Answer from the drawing. Dimensions are ordinates in mm from the lowest x, y and z of the part. Give positions to 0.01 mm unless a question says otherwise; leave off trailing zeros. Loops run counter-clockwise (first coordinate to the right, second up) from the corner with the lowest first, then second, coordinate; pieces in that order, holes last. Notation, with made-up numbers: M 26,-32 L 53,-32 A10 cw 53,-25 Z; hole C -1.75,-36.5 d10. An arc over 180 degrees is marked long. Use a Markdown table: item, result.
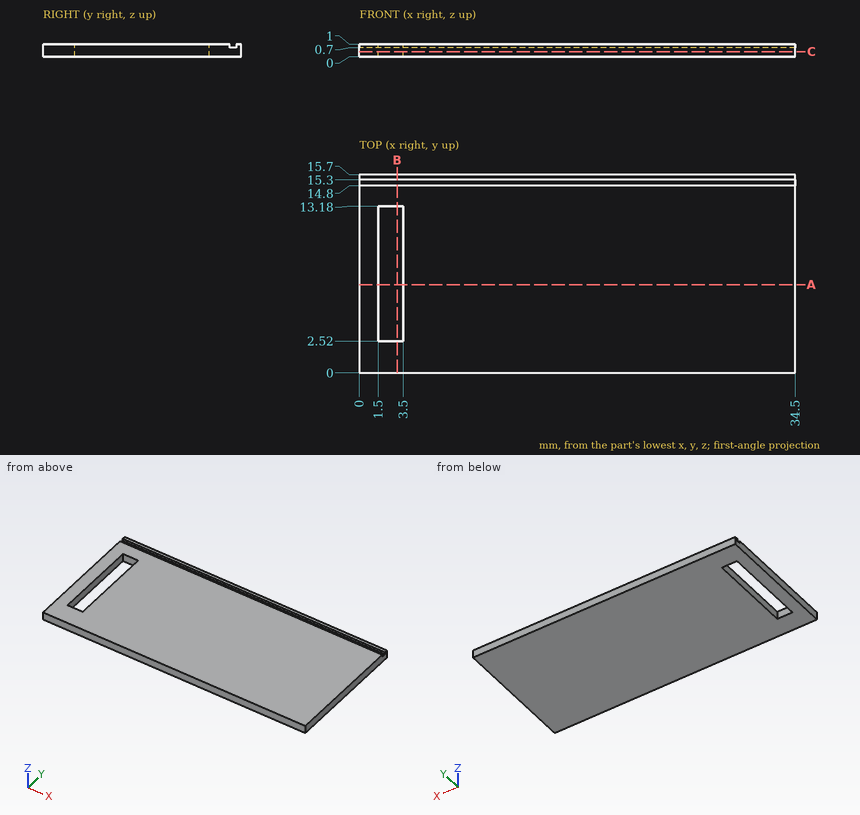
(1) Consider probe 1 along X at (y, z) = (4, 0.4); probe 2 along Y at (x, z) = (33.5, 0.85); probe 3 along Z at (x, y) = (22.5, 15). Determine where each line is inside the solid, lowest interval first. Write a range as [from, to].
Entries:
| item | result |
|---|---|
| probe 1 | x = [0, 1.5], [3.5, 34.5] |
| probe 2 | y = [0, 14.8], [15.3, 15.7] |
| probe 3 | z = [0, 0.7] |
(2) A cutting plane is placed at C-C (z = 0.4). Write down the section's boundary in (x, y), and give its area (3 significant figures).
Entries:
| item | result |
|---|---|
| outline | M 0,0 L 34.5,0 L 34.5,15.7 L 0,15.7 Z; hole M 1.5,2.52 L 3.5,2.52 L 3.5,13.18 L 1.5,13.18 Z |
| area | 520 mm² |
(3) Given P1, Ø8, axis at x = 24.5, y = 3.5, coming from the -Z side, flat-ended and moving along its own axis, determine where the tip first touches the part or whether it passes through.
Entries:
| item | result |
|---|---|
| P1 | stops at z = 0 |
(4) A cutting plane is placed at B-B (x = 3). Write down the section's boundary in (y, z), and give its area (3 significant figures).
Entries:
| item | result |
|---|---|
| outline | M 0,0 L 2.52,0 L 2.52,1 L 0,1 Z; M 13.18,0 L 15.7,0 L 15.7,1 L 15.3,1 L 15.3,0.7 L 14.8,0.7 L 14.8,1 L 13.18,1 Z |
| area | 4.89 mm² |
(5) A cutting plane is placed at A-A (y = 7). Write down the section's boundary in (x, z).
Entries:
| item | result |
|---|---|
| outline | M 0,0 L 1.5,0 L 1.5,1 L 0,1 Z; M 3.5,0 L 34.5,0 L 34.5,1 L 3.5,1 Z |
